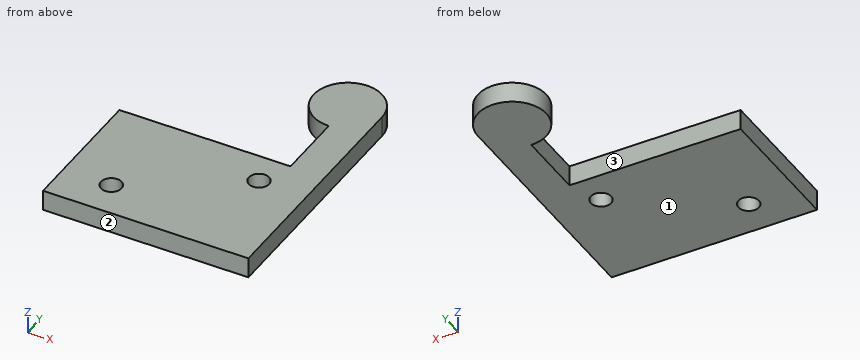
from build123d import *

# Parameters (mm, degrees)
EXTRUDE_1_DEPTH     = 3
SKETCH_2_R          = 1.5
CUT_EXTRUDE_2_DEPTH = 6


with BuildPart() as part:
    # 草图1 → 凸台-拉伸1 (new body)
    with BuildSketch(Plane.XY):
        with BuildLine():
            Line((14.91008261, 4.671258051), (14.91008261, 14.671258051))
            ThreePointArc((14.91008261, 14.671258051), (11.374548704, 23.206791957), (19.91008261, 19.671258051))
            Line((19.91008261, 19.671258051), (19.91008261, 7.339136796))
            Line((19.91008261, 7.339136796), (19.91008261, -15.328741949))
            Line((19.91008261, -15.328741949), (-10.08991739, -15.328741949))
            Line((-10.08991739, -15.328741949), (-10.08991739, 4.671258051))
            Line((-10.08991739, 4.671258051), (14.91008261, 4.671258051))
        make_face()
    extrude(amount=EXTRUDE_1_DEPTH)

    # 草图2 → 切除-拉伸2 (cut)
    with BuildSketch(Plane.XY.offset(3)):
        with Locations((12.91008261, 0)):
            Circle(SKETCH_2_R)
        with Locations((-3.08991739, -10)):
            Circle(SKETCH_2_R)
    extrude(amount=-CUT_EXTRUDE_2_DEPTH, mode=Mode.SUBTRACT)


solid = part.part
Work out the finished part from the listing and answer in its coordinate system (mm). Face numbers are marked on the shaded views. Round coordinates to 2 decimals unless told otherwise and drop trailing zeros. Loops run counter-clockwise (first coordinate to the right, second up) from the corner with the lowest first, then second, coordinate; pieces in that order, holes last. Notation, with made-up numbers: (69, 51) - (111, 51) arc R25 ccw to (111, 75) - close; hole circle Ø3 at (58, 85.5). An arc over 180 degrees is marked (long way). Use one line per item in the form item = value. Start each with the question number.
(1) Consider line 1 (Y direction, x = -3, z = 0.9); line 2 (X direction, y = 14, z = 1.5); line 3 (Y direction, x = 12.25, z = 2.65). Determine where each line is inside the solid, lowest interval first.
(2) Find section D-D on x = 1. Determine the outline of the cut face in (y, z).
(3) Flat-ended cylindrical pins translate along their axes: P1, Ø0.9, axis at y = 8.5, z = 2, coming from the -X side; P2, Ø10, axis at x = 11.5, y = -8, coming from the -Z side; P3, Ø0.9, axis at x = 4.5, z = 1.5, coming from the +Y side. Find the tip coordinate at first contact, or state that the pin passes through.
(4) Determine the mould class of the marked faces 1, 2 and 3 for opening direction Y: +Y half, -Y half, draft (parallel to the pull), parting line (faces both ways), or undercut.
(5) Find section C-C on x = 10.5. Determine the outline of the cut face in (y, z).
(6) Find section B-B on z = 1.4. Determine the outline of the cut face in (x, y), and give its area (3 significant figures).
(7) Find section A-A on y = -10. Determine the outline of the cut face in (x, z).
Answer list:
q1.line_1 = -15.33 to -11.5, -8.5 to 4.67
q1.line_2 = 14.91 to 19.91
q1.line_3 = -15.33 to -1.35, 1.35 to 4.67, 15.44 to 23.9
q2.outline = (-15.33, 0) - (4.67, 0) - (4.67, 3) - (-15.33, 3) - close
q3.P1 = 14.91
q3.P2 = 0
q3.P3 = 4.67
q4.face_1 = draft
q4.face_2 = -Y half
q4.face_3 = undercut
q5.outline = (-15.33, 0) - (4.67, 0) - (4.67, 3) - (-15.33, 3) - close; (17.32, 0) - (22.03, 0) - (22.03, 3) - (17.32, 3) - close
q6.outline = (-10.09, -15.33) - (19.91, -15.33) - (19.91, 19.67) arc R5 ccw (long way) to (14.91, 14.67) - (14.91, 4.67) - (-10.09, 4.67) - close; hole circle Ø3 at (-3.09, -10); hole circle Ø3 at (12.91, 0)
q6.area = 720 mm^2
q7.outline = (-10.09, 0) - (-4.59, 0) - (-4.59, 3) - (-10.09, 3) - close; (-1.59, 0) - (19.91, 0) - (19.91, 3) - (-1.59, 3) - close
